For this review, use the dimensioned drawing (mm, ordinates from the lowest corner) and the shaded views. Give positions to 0.01 mm unless a question says otherwise; leave off trailing zeros. Order: outer loops, then holes, each group sorted by start corner. A loop starts at its lowest first (then second) coordinate and runs counter-clockwise, first axis right, second up.
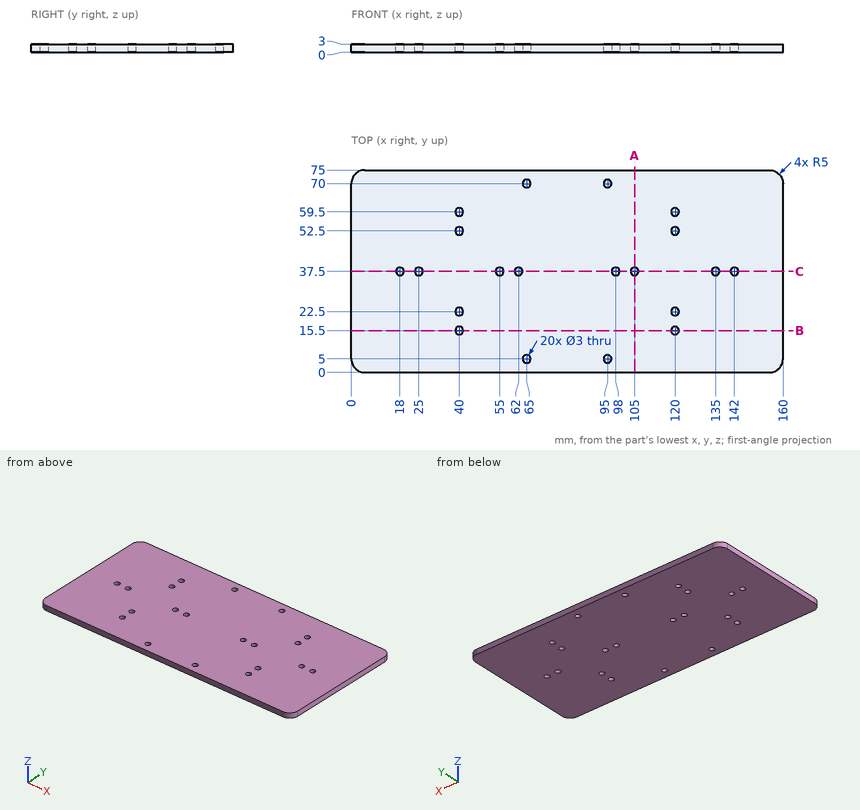
1. Take a section at B-B (y = 15.5). State the section outline as (x, z) points.
Recorded:
outline: (0, 0) - (38.5, 0) - (38.5, 3) - (0, 3) - close; (41.5, 0) - (118.5, 0) - (118.5, 3) - (41.5, 3) - close; (121.5, 0) - (160, 0) - (160, 3) - (121.5, 3) - close
2. For pin 1 (3.5 mm diameter, centred on x = 25, y = 37.5, fed in from +Z), flat-tipped, find the tip position at first contact; note if it passes through.
Recorded:
pin 1: stops at z = 3
3. Take a section at C-C (y = 37.5). State how many separate pieces and enclosed holes the cut face has, then the cut area to 3 significant figures.
Recorded:
separate pieces: 9
enclosed holes: 0
area: 408 mm2
4. Take a section at A-A (x = 105). State the section outline as (y, z) points.
Recorded:
outline: (0, 0) - (36, 0) - (36, 3) - (0, 3) - close; (39, 0) - (75, 0) - (75, 3) - (39, 3) - close
5. For line 1 along Y through (x, z) = (120, 2); line 2 along X through (y, z) = (15.5, 1.65); line 3 along X through (y, z) = (5, 1.1), list the stretches that pass through material, from the lowest coordinate up.
Recorded:
line 1: y = 0 to 14, 17 to 21, 24 to 51, 54 to 58, 61 to 75
line 2: x = 0 to 38.5, 41.5 to 118.5, 121.5 to 160
line 3: x = 0 to 63.5, 66.5 to 93.5, 96.5 to 160
